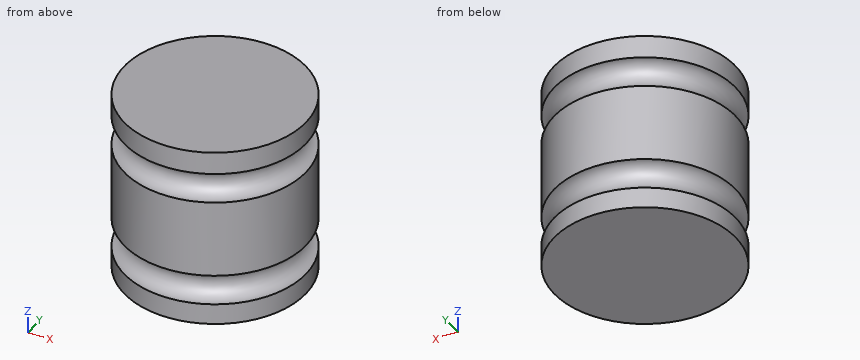
```python
from build123d import *


with BuildPart() as f1:
    # F0 (on Front) → F1 (revolve)
    with BuildSketch(Plane.XZ):
        with BuildLine():
            Line((-38.1, 0), (0, 0))
            Line((0, 0), (0, 8.735418))
            ThreePointArc((0, 8.735418), (-6.35, 15.085418), (0, 21.435418))
            Line((0, 21.435418), (0, 53.991671))
            ThreePointArc((0, 53.991671), (-6.35, 60.341671), (0, 66.691671))
            Line((0, 66.691671), (0, 76.190904))
            Line((0, 76.190904), (-38.1, 76.190904))
            Line((-38.1, 76.190904), (-38.1, 0))
        make_face()
    revolve(axis=Axis((-38.1, 0, 38.095452), (0, 0, 1)))


solid = f1.part
```
Geometry: final body of the model. Coordinates: model frame, mm. Give positions to 0.01 mm unless a question says otherwise; leave off trailing zeros. Write each loop counter-clockwise with the first axis right and the second up, starting at its lowest first coordinate (ties: lowest second). Pieces come first, ordered by that corner, then holes.
1. Section query C-C, the plane z = 46. Return loops of the section in (x, y).
2. Section query A-A, the plane y = 0. Return loops of the section in (x, z), then the cut area to 3 significant figures.
3. Section query D-D, the plane z = 60.5. Return loops of the section in (x, y), then the cut area to 3 significant figures.
4. Section query B-B, the plane x = -38.1. Return loops of the section in (y, z), then the cut area to 3 significant figures.
5. Line query: probe 1 along Z at (x, y) = (-71, -16); probe 2 along Z at (x, y) = (-11.5, 21.5); probe 3 along Y at (x, z) = (-32, 46). Output: solid intervals per line, ascending.
6. Pin query (flat end, axial travel): P1, Ø8, axis at y = -23, z = 19, coming from the +X side; P2, Ø5, axis at y = 20, z = 48, coming from the +X side; P3, Ø12, axis at y = -18.5, z = 14, coming from the +X side. Return the tip coordinate at first contact, or that it passes through.
Computed:
1. outline: circle Ø76.2 at (-38.1, 0)
2. outline: (-76.2, 0) - (0, 0) - (0, 8.74) arc R6.35 cw to (0, 21.44) - (0, 53.99) arc R6.35 cw to (0, 66.69) - (0, 76.19) - (-76.2, 76.19) - (-76.2, 66.69) arc R6.35 cw to (-76.2, 53.99) - (-76.2, 21.44) arc R6.35 cw to (-76.2, 8.74) - close
2. area: 5,550 mm2
3. outline: circle Ø63.5 at (-38.1, 0)
3. area: 3,170 mm2
4. outline: (-38.1, 0) - (38.1, 0) - (38.1, 8.74) arc R6.35 cw to (38.1, 21.44) - (38.1, 53.99) arc R6.35 cw to (38.1, 66.69) - (38.1, 76.19) - (-38.1, 76.19) - (-38.1, 66.69) arc R6.35 cw to (-38.1, 53.99) - (-38.1, 21.44) arc R6.35 cw to (-38.1, 8.74) - close
4. area: 5,550 mm2
5. probe 1: z = 0 to 8.92, 21.25 to 54.18, 66.51 to 76.19
5. probe 2: z = 0 to 10.07, 20.1 to 55.33, 65.35 to 76.19
5. probe 3: y = -37.61 to 37.61
6. P1: stops at x = -5.57
6. P2: stops at x = -4.26
6. P3: stops at x = -3.35
